Build history of the part. All positions in model axes, mm. Face numbers are marked on the shaded views. A direction names the side the tool comes from. Give positions to 0.01 mm unless a question says otherwise; leave off trailing zeros. Loops run counter-clockwise (first coordinate to the right, second up) from the corner with the lowest first, then second, coordinate; pieces in that order, holes last.
1) Two-plate mould, pull along Y, no slides. Class the marked faces 1, 2 and 3: +Y half, -Y half, draft (parallel to the pull), parting line (faces both ways), or undercut.
2) Band-saw the part on D-D on x = 10.75. List the corners of the cut face in (y, z) (3 decimals).
3) 3-axis set-ups, long thin cutter, end or side, ignore diameter. For the marked faces 4, 5 and 6: which of +Z, -Z, +X, -X, +Y, -Y reach the whole face in a straight line?
4) Flat gauge pins, fed straight in: P1, Ø3, axis at x = 13, y = -1.5, coming from the -Z side (3 decimals); P2, Ø1, axis at x = 13.5, z = 1, coming from the -Y side; P3, Ø1.5, axis at x = 11.5, y = 4, coming from the -Z side. Where does each tip first touch, or does it go through?
5) Band-saw the part on C-C on z = 3.25. List the corners of the cut face in (x, y).
6) Wall check: line 1 (X direction, y = 8, z = -5.5); line 2 (Y direction, x = 5.75, z = 0); line 3 (Z direction, x = 8.25, y = 0) (3 decimals). Give the ranges that are in metal, low to high.
7) Band-saw the part on A-A on z = 0. List the corners of the cut face in (x, y) (3 decimals).
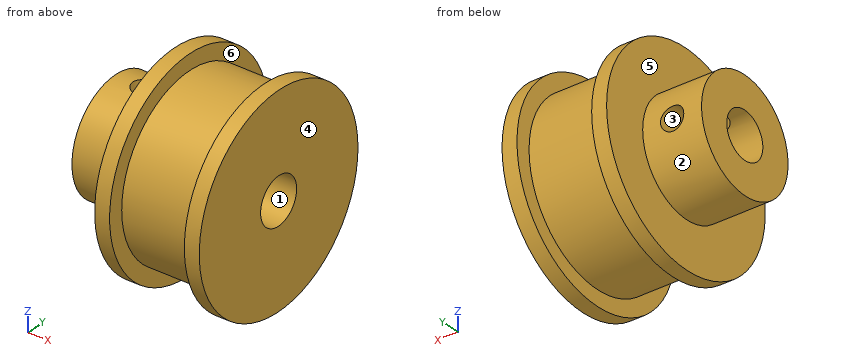
```python
from build123d import *

# Parameters (mm, degrees)
SKETCH2_W = 1.25
SKETCH2_H = 11
SKETCH4_W = 1.25
SKETCH4_H = 11


with BuildPart() as part:
    # Sketch1 → Revolve1 (revolve)
    with BuildSketch(Plane.XY):
        Polygon((0, 2.5), (0, 6), (6.3, 6), (6.3, 11), (7.9, 11), (7.9, 9.325), (15.9, 9.325), (15.9, 11), (17.5, 11), (17.5, 2.5), align=None)
    revolve(axis=Axis((0, 0, 0), (-1, 0, 0)))

    # Sketch2 → M3x0.5 Tapped Hole1 (revolve, cut)
    with BuildSketch(Plane(origin=(3.15, 0, 0), x_dir=(0, 0, -1), z_dir=(1, 0, 0))):
        with Locations((0.625, 5.5)):
            Rectangle(SKETCH2_W, SKETCH2_H)
    revolve(axis=Axis((3.15, -6.35, 0), (0, 1, 0)), mode=Mode.SUBTRACT)

    # Sketch4 → M3x0.5 Tapped Hole2 (revolve, cut)
    with BuildSketch(Plane.YZ.offset(3.15)):
        with Locations((0.625, 5.5)):
            Rectangle(SKETCH4_W, SKETCH4_H)
    revolve(axis=Axis((3.15, 0, -6.35), (0, 0, 1)), mode=Mode.SUBTRACT)


solid = part.part
```
Findings below:
1. face 1: undercut
1. face 2: parting line
1. face 3: draft
2. outline: circle Ø18.65 at (0, 0); hole circle Ø5 at (0, 0)
3. face 4: +Z, -Z, +X, +Y, -Y
3. face 5: -X
3. face 6: none
4. P1: stops at z = -9.325
4. P2: stops at y = -9.31
4. P3: stops at z = -8.74
5. outline: (0, -5.04) - (6.3, -5.04) - (6.3, -10.51) - (7.9, -10.51) - (7.9, -8.74) - (15.9, -8.74) - (15.9, -10.51) - (17.5, -10.51) - (17.5, 10.51) - (15.9, 10.51) - (15.9, 8.74) - (7.9, 8.74) - (7.9, 10.51) - (6.3, 10.51) - (6.3, 5.04) - (0, 5.04) - close; hole circle Ø2.5 at (3.15, 0)
6. line 1: x = 6.3 to 7.9, 15.9 to 17.5
6. line 2: y = -6 to -2.5, 2.5 to 6
6. line 3: z = -9.325 to -2.5, 2.5 to 9.325
7. outline: (0, -6) - (6.3, -6) - (6.3, -11) - (7.9, -11) - (7.9, -9.325) - (15.9, -9.325) - (15.9, -11) - (17.5, -11) - (17.5, -2.5) - (0, -2.5) - close; (0, 2.5) - (1.9, 2.5) - (1.9, 6) - (0, 6) - close; (4.4, 2.5) - (17.5, 2.5) - (17.5, 11) - (15.9, 11) - (15.9, 9.325) - (7.9, 9.325) - (7.9, 11) - (6.3, 11) - (6.3, 6) - (4.4, 6) - close
